Check sheet for the modelled part. Datum: model origin and axes. Units: mm. A direction names the side the tool comes from. Give positions to 0.01 mm unless a question says otherwise; leave off trailing zeros. Write each loop counter-clockwise with the first axis right and the second up, starting at its lowest first coordinate (ties: lowest second). Pieces come first, ordered by that corner, then holes. Notation, with made-up numbers: M 15.25,-40 L 38.25,-40 A13 cw 38.25,-24 Z; hole C 13.5,-24.5 d6. An arc over 180 degrees is marked long. One line per item, written item: value. Start each with the question number.
from build123d import *

# Parameters (mm, degrees)
F1_R     = 43.815
F1_R_2   = 41.275
F2_DEPTH = 101.6
F3_DEPTH = 2.54
F4_R     = 3.81
F5_DEPTH = 57.658
F6_R     = 5.08


# Not quite as in the source:
# - a variable given as a bare number and used for a length is read in inches; the dataset says mm whatever the document's units were


with BuildPart() as f2:
    # F1 (on Top) → F2 (new body)
    with BuildSketch(Plane.XY):
        Circle(F1_R)
        Circle(F1_R_2, mode=Mode.SUBTRACT)
    extrude(amount=F2_DEPTH)

    # F1 (on Top) → F3 (join)
    with BuildSketch(Plane.XY):
        Circle(F1_R_2)
    extrude(amount=F3_DEPTH)

    # F4 (on Front) → F5 (cut, symmetric)
    with BuildSketch(Plane.XZ):
        with Locations((0, 92.71)):
            Circle(F4_R)
        with BuildLine():
            Line((46.664010312, 104.1751918972), (-46.664010312, 104.1751918972))
            Line((-46.664010312, 104.1751918972), (-46.664010312, 86.36))
            Line((-46.664010312, 86.36), (-10.9050826158, 86.36))
            Line((-10.9050826158, 86.36), (-8.5870805957, 95.010901311))
            ThreePointArc((-8.5870805957, 95.010901311), (0, 101.6), (8.5870805957, 95.010901311))
            Line((8.5870805957, 95.010901311), (10.9050826158, 86.36))
            Line((10.9050826158, 86.36), (46.664010312, 86.36))
            Line((46.664010312, 86.36), (46.664010312, 104.1751918972))
        make_face()
    extrude(amount=F5_DEPTH, both=True, mode=Mode.SUBTRACT)

    # F6
    f6_edges = [f2.edges().sort_by_distance(p)[0] for p in [
        (10.905083, -41.122289, 86.36),
        (10.905083, 41.122289, 86.36),
        (-10.905083, -41.122289, 86.36),
        (-10.905083, 41.122289, 86.36),
    ]]
    fillet(f6_edges, radius=F6_R)


solid = f2.part
1) Cross-section at B-B (y = 0). Record the boundary of the cut face in (x, z) (3 decimals).
2) Cross-section at A-A (x = 0). Record the boundary of the cut face in (y, z) (3 decimals), plus the area to 3 significant figures.
3) Tool access check on faces 4 (the cylindrical face through (-5.373, 40.924, 51.38)), 5 (the flat face through (9.232, 41.498, 92.602)). Record the directions out of +Z, -Z, +X, -X, +Y, -Y that give a thin tool (end or side, any length) a straight path to the whole face; none if there is none.
4) Cross-section at D-D (x = -18.5). Record the boundary of the cut face in (y, z).
5) Material ranges on L1, parallel to Y at x = 0, z = 42 (3 decimals); L2, parallel to Z at x = 0, y = -42; L3, parallel to Z at x = -32, y = -22, recorded low to high. Write a range as from..to.
6) Gauge pin test, flat ends, axial feed: pin 1 (25 mm diameter, centred on x = 18, y = 19, fed in from +Z); pin 2 (4.5 mm diameter, centred on x = 0, z = 92.71, fed in from +Y); pin 3 (1 mm diameter, centred on x = -8.5, z = 47, fed in from +Y); pin 4 (4 mm diameter, centred on y = -11, z = 73.5, fed in from -X). Record the tip position at first contact, or that the pin passes through.
7) Cross-section at C-C (z = 92.71). Record the boundary of the cut face in (x, y) (3 decimals), plus the area to 3 significant figures.
8) Draft check along Z on faces 1 (the cylindrical face through (-5.704, 43.442, 50.092)), 2 (the flat face through (41, 6, 86.36)), 3 (the cylindrical face through (-0.496, -42.435, 96.488)). Enter one of: released by +Z, released by -Z, zero draft, split by the parting line, or undercut.
Data:
1. outline: M -43.815,0 L 43.815,0 L 43.815,86.36 L 41.275,86.36 L 41.275,2.54 L -41.275,2.54 L -41.275,86.36 L -43.815,86.36 Z
2. outline: M -43.815,0 L 43.815,0 L 43.815,88.9 L 41.275,88.9 L 41.275,2.54 L -41.275,2.54 L -41.275,88.9 L -43.815,88.9 Z; M -43.815,96.52 L -41.275,96.52 L -41.275,101.6 L -43.815,101.6 Z; M 41.275,96.52 L 43.815,96.52 L 43.815,101.6 L 41.275,101.6 Z
2. area: 687 mm2
3. face 4: +Z
3. face 5: +Z, +X, +Y, -Y
4. outline: M -39.72,0 L 39.72,0 L 39.72,86.36 L 36.9,86.36 L 36.9,2.54 L -36.9,2.54 L -36.9,86.36 L -39.72,86.36 Z
5. L1: y = -43.815..-41.275, 41.275..43.815
5. L2: z = 0..88.9, 96.52..101.6
5. L3: z = 0..2.54
6. pin 1: stops at z = 2.54
6. pin 2: passes through
6. pin 3: stops at y = 43.08
6. pin 4: stops at x = -42.88
7. outline: M -9.204,-42.837 A43.815 ccw -3.81,-43.649 L -3.81,-41.099 A41.275 cw -9.204,-40.236 Z; M -9.204,40.236 A41.275 cw -3.81,41.099 L -3.81,43.649 A43.815 ccw -9.204,42.837 Z; M 3.81,-43.649 A43.815 ccw 9.204,-42.837 L 9.204,-40.236 A41.275 cw 3.81,-41.099 Z; M 3.81,41.099 A41.275 cw 9.204,40.236 L 9.204,42.837 A43.815 ccw 3.81,43.649 Z
7. area: 55.5 mm2
8. face 1: zero draft
8. face 2: released by +Z
8. face 3: undercut
